Autodesk Inventor part; units mm, degrees
ref_plane "YZ Plane" through (0, 0, 0) normal (1, 0, 0) x (0, 1, 0)
ref_plane "XZ Plane" through (0, 0, 0) normal (0, 1, 0) x (-1, 0, 0)
ref_plane "XY Plane" through (0, 0, 0) normal (0, 0, 1) x (1, 0, 0)
sketch "Sketch1" plane through (0, 0, 0) normal (0, 0, 1) x (1, 0, 0)
  arc A0 (20.6801, 49.5146) -> (61.9551, 49.5146) centre (41.3176, 49.5146) ccw
  line L0 (3.2176, 49.5146) -> (79.4176, 49.5146)
  line L1 (3.2176, 49.5146) -> (3.2176, 17.7646)
  line L2 (79.4176, 49.5146) -> (79.4176, 17.7646)
  line L3 (79.4176, 17.7646) -> (3.2176, 17.7646)
  dimension "d21" = 31.75
  dimension "d22" = 31.75
extrude "Extrusion4" add sketch "Sketch1" along normal blind 12.7 contours A0 L0 L2 L3 L1
sketch "Sketch2" plane through (79.4176, 17.7646, 0) normal (1, 0, 0) x (0, 0, -1)
  line L0 (0, 31.75) -> (-12.7, 31.75)
  circle A0 centre (-6.35, 17.4498) radius 3.175
  point P0 (0, -17.7646)
  dimension "d26" = 6.35
extrude "Extrusion5" cut sketch "Sketch2" against normal blind 96.8375
properties part number "Frame Bottom"
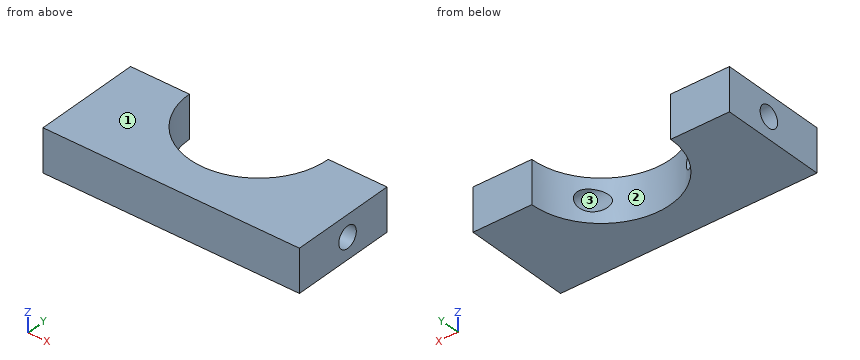
The listing builds one solid part. Answer for the finished solid, in the listing's coordinates (mm). Face numbers are marked on the shaded views. Coordinates: 2 decimals unless noted, no trailing zeros. Order: outer loops, then holes, each group sorted by start corner. A loop starts at its lowest first (then second) coordinate and runs counter-clockwise, first axis right, second up. Notation, with made-up numbers: M 72.25,-3.75 L 91.25,-3.75 A18 ccw 91.25,2.25 Z; hole C 33.25,5 d1. An arc over 180 degrees is marked long. Use CSV: the item, a comma, the result in double quotes.
Q1. Given pin 1 Ø4 at (x, y) = (43, 31.5) entering from -Z, flat-ended and moving along its own axis, determine where the tip first touches the part or whether it passes through.
Here are the results:
pin 1,"through"
Q2. Straight lines are drawn through the part: L1, parallel to Y at x = 9.5, z = 6.35; L2, parallel to X at y = 44, z = 9; L3, parallel to X at y = 41.5, z = 7.5. For each, find the intervals that lie inside material, in ascending order.
Here are the results:
L1,"17.76 to 32.04, 38.39 to 49.51"
L2,"3.22 to 21.43, 61.2 to 79.42"
L3,"3.22 to 22.3, 60.34 to 79.42"
Q3. Section A-A (z = 6.35) is taken. Determine the outline of the cut face in (x, y) (1 decimal).
Here are the results:
outline,"M 3.2,17.8 L 79.4,17.8 L 79.4,32 L 52.3,32 A20.6 cw 30.3,32 L 3.2,32 Z; M 3.2,38.4 L 23.9,38.4 A20.6 cw 20.7,49.5 L 3.2,49.5 Z; M 58.7,38.4 L 79.4,38.4 L 79.4,49.5 L 62,49.5 A20.6 cw Z"
Q4. Section B-B (y = 34) is taken. Determine the outline of the cut face in (x, z), then the cut area to 3 significant figures.
Here are the results:
outline,"M 3.22,0 L 27.71,0 L 27.71,3.42 L 3.22,3.42 Z; M 3.22,9.28 L 27.71,9.28 L 27.71,12.7 L 3.22,12.7 Z; M 54.93,0 L 79.42,0 L 79.42,3.42 L 54.93,3.42 Z; M 54.93,9.28 L 79.42,9.28 L 79.42,12.7 L 54.93,12.7 Z"
area,"335 mm2"
Q5. Determine the mould class of the marked faces 1, 2 and 3 for opening direction Y: pulls with the +Y half, pulls with the -Y half, needs draft (parallel to the pull), parting line crosses it, or undercut.
Here are the results:
face 1,"needs draft"
face 2,"pulls with the +Y half"
face 3,"undercut"
Q6. Section C-C (x = 9.5) is taken. Determine the outline of the cut face in (y, z) (3 decimals).
Here are the results:
outline,"M 17.765,0 L 49.515,0 L 49.515,12.7 L 17.765,12.7 Z; hole C 35.214,6.35 d6.35"
Q7. Section D-D (y = 44) is taken. Determine the outline of the cut face in (x, z), then the cut area to 3 significant figures.
Here are the results:
outline,"M 3.22,0 L 21.43,0 L 21.43,12.7 L 3.22,12.7 Z; M 61.2,0 L 79.42,0 L 79.42,12.7 L 61.2,12.7 Z"
area,"463 mm2"
